```python
from build123d import *

# Parameters (mm, degrees)
F0_W     = 66.167
F0_H     = 12.7
F0_W_2   = 194.183
F0_W_3   = 19.05
F3_DEPTH = 2.54
F4_DEPTH = 25.4


with BuildPart() as f1:
    # F0 (on Front) → F1 (revolve)
    with BuildSketch(Plane.XZ):
        with Locations((33.0835, 6.35)):
            Rectangle(F0_W, F0_H)
        with Locations((163.2585, 6.35)):
            Rectangle(F0_W_2, F0_H)
        with Locations((269.875, 6.35)):
            Rectangle(F0_W_3, F0_H)
    revolve(axis=Axis((155.896521, 0, 0), (1, 0, 0)))

    # F2 (on face) → F3 (cut)
    with BuildSketch(Plane.YZ.offset(279.4)):
        with BuildLine():
            ThreePointArc((-2.54, 5.819871), (0, 6.35), (2.54, 5.819871))
            Line((2.54, 5.819871), (2.54, 12.443408))
            ThreePointArc((2.54, 12.443408), (0, 12.7), (-2.54, 12.443408))
            Line((-2.54, 12.443408), (-2.54, 5.819871))
        make_face()
        with BuildLine():
            ThreePointArc((-5.819871, -2.54), (-6.35, 0), (-5.819871, 2.54))
            Line((-5.819871, 2.54), (-12.443408, 2.54))
            ThreePointArc((-12.443408, 2.54), (-12.7, 0), (-12.443408, -2.54))
            Line((-12.443408, -2.54), (-5.819871, -2.54))
        make_face()
        with BuildLine():
            Line((2.54, -12.443408), (2.54, -5.819871))
            ThreePointArc((2.54, -5.819871), (0, -6.35), (-2.54, -5.819871))
            Line((-2.54, -5.819871), (-2.54, -12.443408))
            ThreePointArc((-2.54, -12.443408), (0, -12.7), (2.54, -12.443408))
        make_face()
        with BuildLine():
            ThreePointArc((5.819871, 2.54), (6.216055, 1.297366), (6.35, 0))
            ThreePointArc((6.35, 0), (6.216055, -1.297366), (5.819871, -2.54))
            Line((5.819871, -2.54), (12.443408, -2.54))
            ThreePointArc((12.443408, -2.54), (12.635689, -1.276464), (12.7, 0))
            ThreePointArc((12.7, 0), (12.635689, 1.276464), (12.443408, 2.54))
            Line((12.443408, 2.54), (5.819871, 2.54))
        make_face()
    extrude(amount=-F3_DEPTH, mode=Mode.SUBTRACT)

    # F2 (on face) → F4 (cut)
    with BuildSketch(Plane.YZ.offset(279.4)):
        with BuildLine():
            ThreePointArc((5.819871, -2.54), (6.216055, -1.297366), (6.35, 0))
            ThreePointArc((6.35, 0), (6.216055, 1.297366), (5.819871, 2.54))
            ThreePointArc((5.819871, 2.54), (4.490128, 4.490128), (2.54, 5.819871))
            ThreePointArc((2.54, 5.819871), (0, 6.35), (-2.54, 5.819871))
            ThreePointArc((-2.54, 5.819871), (-4.490128, 4.490128), (-5.819871, 2.54))
            ThreePointArc((-5.819871, 2.54), (-6.35, 0), (-5.819871, -2.54))
            ThreePointArc((-5.819871, -2.54), (-4.490128, -4.490128), (-2.54, -5.819871))
            ThreePointArc((-2.54, -5.819871), (0, -6.35), (2.54, -5.819871))
            ThreePointArc((2.54, -5.819871), (4.490128, -4.490128), (5.819871, -2.54))
        make_face()
    extrude(amount=-F4_DEPTH, mode=Mode.SUBTRACT)


solid = f1.part
```
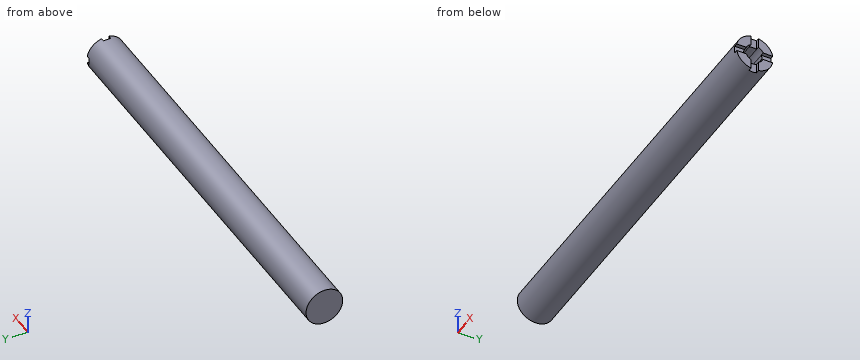
The listing builds one solid part. Answer for the finished solid, in the listing's coordinates (mm). Coordinates: 2 decimals unless noted, no trailing zeros. Loops run counter-clockwise (first coordinate to the right, second up) from the corner with the lowest first, then second, coordinate; pieces in that order, holes last. Notation, with made-up numbers: (-10, 46.25) -> (-3, 46.25) arc R18 cw to (-3, 60.25) -> close; hole circle Ø5 at (19.25, 57.25). An arc over 180 degrees is marked (long way). Use one line per item in the form item = value. Start each with the question number.
Item 1: The part is cut by section B-B on x = 159. Determine the outline of the cut face in (y, z), then the cut area to 3 significant figures.
Item 2: Flat-ended cylindrical pins translate along their axes: pin 1 Ø2.5 at (y, z) = (0, -9.5) entering from +X; pin 2 Ø2 at (x, y) = (278.5, -8.5) entering from +Z; pin 3 Ø1 at (x, z) = (38, -2.5) entering from +Y. Find the tip coordinate at first contact, or state that the pin passes through.
Item 3: The part is cut by section A-A on y = 0. Determine the outline of the cut face in (x, z).
Item 4: Consider L1, parallel to Z at x = 52, y = -0.75; L2, parallel to X at y = -2.75, z = -3.5; L3, parallel to Z at x = 256, y = -3.5. Determine where each line is inside the solid, lowest interval first. Write a range as [from, to].
Answer key:
q1.outline = circle Ø25.4 at (0, 0)
q1.area = 507 mm2
q2.pin_1 = 276.86
q2.pin_2 = 10.25
q2.pin_3 = 12.54
q3.outline = (0, -12.7) -> (276.86, -12.7) -> (276.86, -6.35) -> (254, -6.35) -> (254, 6.35) -> (276.86, 6.35) -> (276.86, 12.7) -> (0, 12.7) -> close
q4.L1 = [-12.68, 12.68]
q4.L2 = [0, 254]
q4.L3 = [-12.21, -5.3], [5.3, 12.21]
